Input: part model. Units: mm. Frame: model coordinates. A direction names the side the tool comes from. Give positions to 0.01 mm unless a question says otherwise; leave off trailing zeros. Write each loop counter-clockwise with the first axis right and the second up, starting at its lowest first coordinate (ties: lowest second). Pieces come first, ordered by that corner, then holes. Notation, with made-up numbers: (-7.5, 2) -> (-2.5, 2) arc R12 cw to (-2.5, 24) -> close; hole circle Ø5 at (37.25, 59). An arc over 180 degrees is marked (long way). Return JSON: item names as keys, results as strings. Group by question number.
Item 1: Mould query, pull axis X, two halves, no side actions, for faces 1 (the face through (-1, 2, 37)), 2 (the face through (41.78, 0.16, 32.94)), 3 (the face through (53, 3, 18)). Classes: released by +X, released by -X, zero draft, split by the parting line, or undercut.
Item 2: Set-up query: faces 4 (the face through (-44.22, 0.16, 32.94)), 5 (the face through (41.78, -0.16, 4.46)), 6 (the face through (-52, -2, 19)). Return all of +Z, -Z, +X, -X, +Y, -Y with unobstructed straight access to the full face (end or side cutting, diameter ignored); none if empty.
Item 3: Section A-A, the plane z = 4. Return loops of the section in (x, y).
Item 4: Pin query (flat end, axial travel): P1, Ø1.5, axis at x = 43, y = 0, coming from the +Z side; P2, Ø1.5, axis at x = 43, y = 0, coming from the -Z side; P3, Ø1, axis at y = -0.5, z = 24, coming from the +X side. Return the tip coordinate at first contact, or that it passes through.
Item 5: Line query: line 1 (Y direction, x = 43, z = 32); line 2 (X direction, y = 0, z = 35.75); line 3 (X direction, y = -0.5, z = 2). Output: solid intervals per line, ascending. Write a range as [from, to].
Autodesk Inventor part; units mm, degrees
ref_plane "YZ Plane" through (0, 0, 0) normal (1, 0, 0) x (0, 1, 0)
ref_plane "XZ Plane" through (0, 0, 0) normal (0, 1, 0) x (-1, 0, 0)
ref_plane "XY Plane" through (0, 0, 0) normal (0, 0, 1) x (1, 0, 0)
sketch "Sketch1" plane through (0, 0, 0) normal (0, 0, 1) x (1, 0, 0)
  line L0 (-53, 4) -> (53, 4)
  line L1 (53, 4) -> (53, -4)
  line L2 (53, -4) -> (-53, -4)
  line L3 (-53, -4) -> (-53, 4)
  line L4 (-53, 4) -> (53, -4) construction
  line L5 (53, 4) -> (-53, -4) construction
  point P0 (0, 0)
  dimension "d0" = 106
  dimension "d1" = 8
extrude "Extrusion1" add sketch "Sketch1" along normal blind 37
sketch "Sketch2" plane through (0, 0, 37) normal (0, 0, 1) x (1, 0, 0)
  line L0 (-53, 4) -> (-53, -4)
  line L1 (53, -4) -> (53, 4)
  point P0 (0, 0)
  point P1 (-43, 0)
  point P2 (0, 0)
  point P3 (43, 0)
  dimension "d4" = 10
  dimension "d5" = 10
hole "Hole1" at (-43, 0, 37) at (0, 0, 37) at (43, 0, 37) direction (0, 0, -1) diameter 2.459 depth 8 tip angle 118
sketch "Sketch3" plane through (0, 0, 0) normal (0, 0, -1) x (-1, 0, 0)
  circle A0 centre (43, 0) radius 1.2295
  circle A1 centre (0, 0) radius 1.2295
  circle A2 centre (-43, 0) radius 1.2295
hole "Hole2" at (-43, 0, 0) at (0, 0, 0) at (43, 0, 0) direction (0, 0, 1) diameter 2.459 depth 8.8 tip angle 118
fillet "Fillet1" radius 5 2 edges at (-53, -4, 18.5) (53, -4, 18.5)
sketch "Sketch4" plane through (0, 0, 37) normal (0, 0, 1) x (1, 0, 0)
  point P0 (0, 0)
  point P1 (-25, 0)
  point P2 (25, 0)
  dimension "d21" = 25
  dimension "d22" = 25
hole "Hole3" [suppressed]
sketch "Sketch5" plane through (0, 0, 0) normal (0, 0, -1) x (-1, 0, 0)
  circle A0 centre (25, 0) radius 1.5
  circle A1 centre (-25, 0) radius 1.5
  point P0 (0, 0)
hole "Hole4" [suppressed]
properties part number "side 2" material "Aluminum 6061"
Answer below:
{
 "1": {"face 1": "zero draft", "face 2": "undercut", "face 3": "released by +X"},
 "2": {"face 4": "+Z", "face 5": "-Z", "face 6": "+Z, -Z, -X, -Y"},
 "3": {"outline": "(-53, 1) arc R5 ccw to (-48, -4) -> (48, -4) arc R5 ccw to (53, 1) -> (53, 4) -> (-53, 4) -> close; hole circle Ø2.46 at (-43, 0); hole circle Ø2.46 at (0, 0); hole circle Ø2.46 at (43, 0)"},
 "4": {"P1": "stops at z = 28.71", "P2": "stops at z = 9.09", "P3": "stops at x = 52.9"},
 "5": {"line 1": "y = [-4, -1.23], [1.23, 4]", "line 2": "x = [-52.9, -44.23], [-41.77, -1.23], [1.23, 41.77], [44.23, 52.9]", "line 3": "x = [-52.77, -44.12], [-41.88, -1.12], [1.12, 41.88], [44.12, 52.77]"}
}
